from build123d import *

# Parameters (mm, degrees)
BOSS_EXTRUDE1_DEPTH = 3.175
SKETCH2_R           = 2.5
CUT_EXTRUDE1_DEPTH  = 4.175
BOSS_EXTRUDE2_DEPTH = 3.175
SKETCH4_R           = 2.505
CUT_EXTRUDE2_DEPTH  = 4.175


with BuildPart() as part:
    # Sketch1 → Boss-Extrude1 (new body)
    with BuildSketch(Plane.XY):
        with BuildLine():
            Line((26.334969325, 167.047852761), (23.159969325, 167.047852761))
            Line((23.159969325, 167.047852761), (-21.290030675, 167.047852761))
            ThreePointArc((-21.290030675, 167.047852761), (-23.535094705, 166.117916791), (-24.465030675, 163.872852761))
            Line((-24.465030675, 163.872852761), (-24.465030675, 14.647852761))
            Line((-24.465030675, 14.647852761), (26.334969325, 14.647852761))
            Line((26.334969325, 14.647852761), (26.334969325, 163.872852761))
            Line((26.334969325, 163.872852761), (26.334969325, 167.047852761))
        make_face()
        with BuildLine():
            Line((99.359969325, 14.647852761), (26.334969325, 14.647852761))
            Line((26.334969325, 14.647852761), (-24.465030675, 14.647852761))
            Line((-24.465030675, 14.647852761), (-24.465030675, -32.977147239))
            ThreePointArc((-24.465030675, -32.977147239), (-23.535094705, -35.22221127), (-21.290030675, -36.152147239))
            Line((-21.290030675, -36.152147239), (99.359969325, -36.152147239))
            ThreePointArc((99.359969325, -36.152147239), (101.605033355, -35.22221127), (102.534969325, -32.977147239))
            Line((102.534969325, -32.977147239), (102.534969325, 11.472852761))
            ThreePointArc((102.534969325, 11.472852761), (101.605033355, 13.717916791), (99.359969325, 14.647852761))
        make_face()
    extrude(amount=BOSS_EXTRUDE1_DEPTH)

    # Sketch2 → Cut-Extrude1 (cut, through all)
    with BuildSketch(Plane.XY.offset(3.175)):
        with Locations((-11.765030675, 154.347852761)):
            Circle(SKETCH2_R)
        with Locations((89.834969325, -23.452147239)):
            Circle(SKETCH2_R)
        with Locations((0.934969325, 154.347852761)):
            Circle(SKETCH2_R)
        with Locations((13.634969325, 154.347852761)):
            Circle(SKETCH2_R)
        with Locations((0.934969325, 141.647852761)):
            Circle(SKETCH2_R)
        with Locations((13.634969325, 141.647852761)):
            Circle(SKETCH2_R)
        with Locations((0.934969325, 128.947852761)):
            Circle(SKETCH2_R)
        with Locations((13.634969325, 128.947852761)):
            Circle(SKETCH2_R)
        with Locations((0.934969325, 116.247852761)):
            Circle(SKETCH2_R)
        with Locations((13.634969325, 116.247852761)):
            Circle(SKETCH2_R)
        with Locations((0.934969325, 103.547852761)):
            Circle(SKETCH2_R)
        with Locations((13.634969325, 103.547852761)):
            Circle(SKETCH2_R)
        with Locations((0.934969325, 90.847852761)):
            Circle(SKETCH2_R)
        with Locations((13.634969325, 90.847852761)):
            Circle(SKETCH2_R)
        with Locations((-11.765030675, 141.647852761)):
            Circle(SKETCH2_R)
        with Locations((-11.765030675, 128.947852761)):
            Circle(SKETCH2_R)
        with Locations((-11.765030675, 116.247852761)):
            Circle(SKETCH2_R)
        with Locations((-11.765030675, 103.547852761)):
            Circle(SKETCH2_R)
        with Locations((-11.765030675, 90.847852761)):
            Circle(SKETCH2_R)
        with Locations((77.134969325, -23.452147239)):
            Circle(SKETCH2_R)
        with Locations((64.434969325, -23.452147239)):
            Circle(SKETCH2_R)
        with Locations((51.734969325, -23.452147239)):
            Circle(SKETCH2_R)
        with Locations((39.034969325, -23.452147239)):
            Circle(SKETCH2_R)
        with Locations((77.134969325, -10.752147239)):
            Circle(SKETCH2_R)
        with Locations((64.434969325, -10.752147239)):
            Circle(SKETCH2_R)
        with Locations((51.734969325, -10.752147239)):
            Circle(SKETCH2_R)
        with Locations((39.034969325, -10.752147239)):
            Circle(SKETCH2_R)
        with Locations((77.134969325, 1.947852761)):
            Circle(SKETCH2_R)
        with Locations((64.434969325, 1.947852761)):
            Circle(SKETCH2_R)
        with Locations((51.734969325, 1.947852761)):
            Circle(SKETCH2_R)
        with Locations((39.034969325, 1.947852761)):
            Circle(SKETCH2_R)
        with Locations((89.834969325, -10.752147239)):
            Circle(SKETCH2_R)
        with Locations((89.834969325, 1.947852761)):
            Circle(SKETCH2_R)
        with Locations((-11.765030675, 40.047852761)):
            Circle(SKETCH2_R)
        with Locations((0.934969325, 40.047852761)):
            Circle(SKETCH2_R)
        with Locations((13.634969325, 40.047852761)):
            Circle(SKETCH2_R)
        with Locations((-11.765030675, 27.347852761)):
            Circle(SKETCH2_R)
        with Locations((0.934969325, 27.347852761)):
            Circle(SKETCH2_R)
        with Locations((13.634969325, 27.347852761)):
            Circle(SKETCH2_R)
        with Locations((-11.765030675, 14.647852761)):
            Circle(SKETCH2_R)
        with Locations((0.934969325, 14.647852761)):
            Circle(SKETCH2_R)
        with Locations((13.634969325, 14.647852761)):
            Circle(SKETCH2_R)
        with Locations((-11.765030675, 1.947852761)):
            Circle(SKETCH2_R)
        with Locations((0.934969325, 1.947852761)):
            Circle(SKETCH2_R)
        with Locations((13.634969325, 1.947852761)):
            Circle(SKETCH2_R)
        with Locations((-11.765030675, -10.752147239)):
            Circle(SKETCH2_R)
        with Locations((0.934969325, -10.752147239)):
            Circle(SKETCH2_R)
        with Locations((13.634969325, -10.752147239)):
            Circle(SKETCH2_R)
        with Locations((-11.765030675, -23.452147239)):
            Circle(SKETCH2_R)
        with Locations((0.934969325, -23.452147239)):
            Circle(SKETCH2_R)
        with Locations((13.634969325, -23.452147239)):
            Circle(SKETCH2_R)
    extrude(amount=-CUT_EXTRUDE1_DEPTH, mode=Mode.SUBTRACT)

    # Sketch3 → Boss-Extrude2 (add)
    with BuildSketch(Plane.XY.offset(3.175)):
        with BuildLine():
            Line((73.959969325, 167.047852761), (26.334969325, 167.047852761))
            Line((26.334969325, 167.047852761), (26.334969325, 116.247852761))
            Line((26.334969325, 116.247852761), (73.959969325, 116.247852761))
            ThreePointArc((73.959969325, 116.247852761), (76.205033355, 117.17778873), (77.134969325, 119.422852761))
            Line((77.134969325, 119.422852761), (77.134969325, 163.872852761))
            ThreePointArc((77.134969325, 163.872852761), (76.205033355, 166.117916791), (73.959969325, 167.047852761))
        make_face()
    extrude(amount=-BOSS_EXTRUDE2_DEPTH)

    # Sketch4 → Cut-Extrude2 (cut, through all)
    with BuildSketch(Plane.XY.offset(3.175)):
        with Locations((64.434969325, 154.347852761)):
            Circle(SKETCH4_R)
        with Locations((51.734969325, 154.347852761)):
            Circle(SKETCH4_R)
        with Locations((39.034969325, 154.347852761)):
            Circle(SKETCH4_R)
        with Locations((51.734969325, 141.647852761)):
            Circle(SKETCH4_R)
        with Locations((39.034969325, 141.647852761)):
            Circle(SKETCH4_R)
        with Locations((51.734969325, 128.947852761)):
            Circle(SKETCH4_R)
        with Locations((39.034969325, 128.947852761)):
            Circle(SKETCH4_R)
        with Locations((64.434969325, 141.647852761)):
            Circle(SKETCH4_R)
        with Locations((64.434969325, 128.947852761)):
            Circle(SKETCH4_R)
    extrude(amount=-CUT_EXTRUDE2_DEPTH, mode=Mode.SUBTRACT)


solid = part.part
Source: CAD feature listing. Evaluate the final solid. Frame: model axes, mm. Give positions to 0.01 mm unless a question says otherwise; leave off trailing zeros. Write each loop counter-clockwise with the first axis right and the second up, starting at its lowest first coordinate (ties: lowest second). Pieces come first, ordered by that corner, then holes. Notation, with made-up numbers: (57, -13) -> (64, -13) arc R30 ccw to (64, 17) -> close; hole circle Ø7 at (42.25, -0.5). An arc over 180 degrees is marked (long way). Return JSON: item names as keys, results as strings. Group by question number.
1. Material intervals for line 1 (Y direction, x = 88, z = 2.85); line 2 (Y direction, x = 34, z = 0.25); line 3 (X direction, y = 76.5, z = 0.2), sorted ascending. Write a range as from..to.
2. Section B-B, the plane y = 75.5. Output: boundary loops of the cut face in (x, z) (3 decimals), then the cut area to 3 significant figures.
3. Pin query (flat end, axial travel): pin 1 Ø4 at (x, y) = (-11.77, 154.35) entering from -Z; pin 2 Ø1 at (y, z) = (74, 2.5) entering from +X. Return the tip coordinate at first contact, or that it passes through.
4. Section C-C, the plane x = 14. Count the separate pieces of the cut face and the enclosed holes in it, then the cut area to 3 significant figures.
5. Section A-A, the plane x = 58. Output: boundary loops of the cut face in (y, z) (3 decimals), then the cut area to 3 significant figures.
6. Mould query, pull axis X, two halves, no side actions, for faces 1 (the face through (-10.61, 152.13, 1.61)), 2 (the face through (24, 67, 0)). Classes: +X half, -X half, draft (parallel to the pull), parting line (faces both ways), or undercut.
Determined:
{
 "1": {"line 1": "y = -36.15..-25.15, -21.75..-12.45, -9.05..0.25, 3.65..14.65", "line 2": "y = -36.15..14.65, 116.25..167.05", "line 3": "x = -24.47..26.33"},
 "2": {"outline": "(-24.465, 0) -> (26.335, 0) -> (26.335, 3.175) -> (-24.465, 3.175) -> close", "area": "161 mm2"},
 "3": {"pin 1": "passes through", "pin 2": "stops at x = 26.33"},
 "4": {"separate pieces": "13", "enclosed holes": "0", "area": "457 mm2"},
 "5": {"outline": "(-36.152, 0) -> (14.648, 0) -> (14.648, 3.175) -> (-36.152, 3.175) -> close; (116.248, 0) -> (167.048, 0) -> (167.048, 3.175) -> (116.248, 3.175) -> close", "area": "323 mm2"},
 "6": {"face 1": "undercut", "face 2": "draft"}
}
